Verification items for the finished model (mm, model axes). Face numbers are marked on the shaded views. A direction names the side the tool comes from. Give positions to 0.01 mm unless a question says otherwise; leave off trailing zeros. Write each loop counter-clockwise with the first axis right and the second up, starting at its lowest first coordinate (ties: lowest second). Pieces come first, ordered by that corner, then holes. Notation, with made-up numbers: (81, 23.25) -> (86, 23.25) arc R22 ccw to (86, 29.25) -> close; hole circle Ø6 at (-9.5, 11). An arc over 180 degrees is marked (long way). Answer as CSV lines item,"result". Start each with the question number.
1) Sectioned sample at C-C on y = 18. Record the cut outline in (x, z), and give its area (3 significant figures).
2) Tool access check on the marked faces 5, 6 and 7. Record the directions out of +Z, -Z, +X, -X, +Y, -Y that give a thin tool (end or side, any length) a straight path to the whole face; none if there is none.
3) Gauge pin test, flat ends, axial feed: pin 1 Ø10 at (x, y) = (-4.5, 21) entering from +Z; pin 2 Ø1.5 at (x, z) = (5, 2) entering from +Y; pin 3 Ø9 at (x, y) = (0, 23.5) entering from -Z. Record the tip position at first contact, or that the pin passes through.
4) Mould release check, pull along Z, two halves, no side actions. Record for the marked faces 1, 2, 3 and 4: released by +Z, released by -Z, zero draft, split by the parting line, or undercut.
5) Sectioned sample at B-B on z = 4.5. Record the cut outline in (x, y).
6) Sectioned sample at A-A on y = -0.5. Record the cut outline in (x, z), and give its area (3 significant figures).
7) Material ranges on L1, parallel to Z at x = 3, y = 2.5; L2, parallel to Z at x = -2, y = 41; L3, parallel to Y at x = -11.5, z = 13, recorded low to high.
```python
from build123d import *

# Parameters (mm, degrees)
F0_W     = 31.75
F0_H     = 25.4
F1_DEPTH = 3.81
F2_W     = 31.75
F2_H     = 3.81
F3_DEPTH = 3.81
F5_W     = 31.75
F5_H     = 5.08
F6_DEPTH = 31.75
F7_R     = 8.5850562929
F8_DEPTH = 10.161
F9_R     = 15.875
F10_R    = 15.87499
F11_R    = 1.27
F12_R    = 2.53999


# Not quite as in the source:
# - a fillet or chamfer is up to 0.001 mm smaller than in the source, because OpenCascade refuses the exact size


with BuildPart() as f1:
    # F0 (on Top) → F1 (new body)
    with BuildSketch(Plane.XY):
        with Locations((1.8298272586, 1.9303451554)):
            Rectangle(F0_W, F0_H)
    extrude(amount=F1_DEPTH)

    # F2 (on face) → F3 (join)
    with BuildSketch(Plane.XY.offset(3.81)):
        with Locations((1.8298272586, 12.7253451554)):
            Rectangle(F2_W, F2_H)
    extrude(amount=F3_DEPTH)

    # F4: F1 across face


with BuildPart() as f1_1:
    add(f1.part)
    add(f1.part.mirror(Plane(origin=(1.8298272586, 12.7253451554, 7.62), x_dir=(1, 0, 0), z_dir=(0, 0, 1))))

    # F5 (on face) → F6 (join)
    with BuildSketch(Plane(origin=(0, 14.6303451554, 0), x_dir=(-1, 0, 0), z_dir=(0, 1, 0))):
        with Locations((-1.8298272586, 7.62)):
            Rectangle(F5_W, F5_H)
    extrude(amount=F6_DEPTH)

    # F7 (on face) → F8 (cut, through all)
    with BuildSketch(Plane(origin=(0, 0, 5.08), x_dir=(1, 0, 0), z_dir=(0, 0, -1))):
        with Locations((1.8298272586, -30.5053451554)):
            Circle(F7_R)
    extrude(amount=-F8_DEPTH, mode=Mode.SUBTRACT)

    # F9
    f9_edges = [f1_1.edges().sort_by_distance(p)[0] for p in [
        (17.704827, 46.380345, 7.62),
    ]]
    fillet(f9_edges, radius=F9_R)

    # F10 (radius 15.875 in the source; OpenCascade refuses exactly that, so slightly less here)
    f10_edges = [f1_1.edges().sort_by_distance(p)[0] for p in [
        (-14.045173, 46.380345, 7.62),
    ]]
    fillet(f10_edges, radius=F10_R)

    # F11
    f11_edges = [f1_1.edges().sort_by_distance(p)[0] for p in [
        (-14.045173, -10.769655, 13.335),
        (-14.045173, 0.025345, 11.43),
        (-14.045173, 1.930345, 15.24),
        (-14.045173, 0.025345, 3.81),
        (-14.045173, 1.930345, 0),
        (-14.045173, 10.820345, 7.62),
        (-14.045173, 22.56785, 10.16),
        (-14.045173, 22.56785, 5.08),
        (1.829827, 14.630345, 15.24),
        (-14.045173, 14.630345, 12.7),
        (-14.045173, 14.630345, 2.54),
        (1.829827, -10.769655, 3.81),
        (1.829827, -10.769655, 11.43),
        (1.829827, -10.769655, 0),
        (1.829827, -10.769655, 15.24),
        (17.704827, 1.930345, 15.24),
        (17.704827, 0.025345, 11.43),
        (17.704827, 0.025345, 3.81),
        (17.704827, 1.930345, 0),
        (17.704827, 14.630345, 2.54),
        (17.704827, 14.630345, 12.7),
        (17.704827, 10.820345, 7.62),
    ]]
    fillet(f11_edges, radius=F11_R)

    # F12 (radius 2.54 in the source; OpenCascade refuses exactly that, so slightly less here)
    f12_edges = [f1_1.edges().sort_by_distance(p)[0] for p in [
        (-6.755229, 30.505345, 10.16),
        (-6.755229, 30.505345, 5.08),
    ]]
    fillet(f12_edges, radius=F12_R)


solid = f1_1.part
```
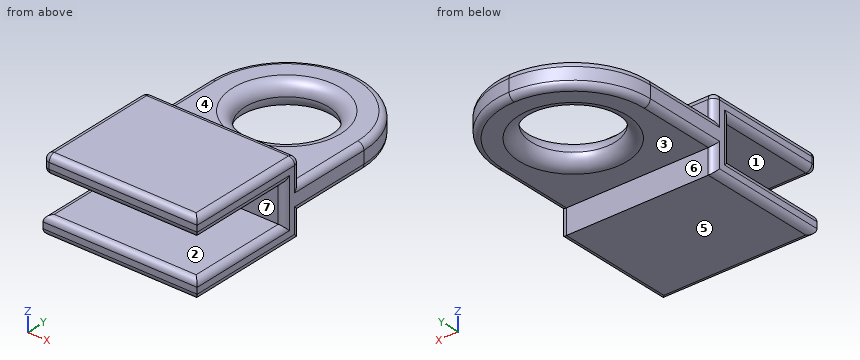
Ans:
1,outline,"(-14.05, 6.35) arc R1.27 ccw to (-12.78, 5.08) -> (16.43, 5.08) arc R1.27 ccw to (17.7, 6.35) -> (17.7, 8.89) arc R1.27 ccw to (16.43, 10.16) -> (-12.78, 10.16) arc R1.27 ccw to (-14.05, 8.89) -> close"
1,area,"160 mm²"
2,face 5,"-Z, +X, -X, +Y, -Y"
2,face 6,"-Z, +X, -X, +Y"
2,face 7,"+X, -X, -Y"
3,pin 1,"stops at z = 10.16"
3,pin 2,"stops at y = 14.63"
3,pin 3,"stops at z = 5.08"
4,face 1,"undercut"
4,face 2,"undercut"
4,face 3,"released by -Z"
4,face 4,"released by +Z"
5,outline,"(-14.05, 12.09) arc R1.27 ccw to (-12.78, 10.82) -> (16.43, 10.82) arc R1.27 ccw to (17.7, 12.09) -> (17.7, 13.36) arc R1.27 ccw to (16.43, 14.63) -> (-12.78, 14.63) arc R1.27 ccw to (-14.05, 13.36) -> close"
6,outline,"(-14.05, 1.27) arc R1.27 ccw to (-12.78, 0) -> (16.43, 0) arc R1.27 ccw to (17.7, 1.27) -> (17.7, 2.54) arc R1.27 ccw to (16.43, 3.81) -> (-12.78, 3.81) arc R1.27 ccw to (-14.05, 2.54) -> close; (-14.05, 12.7) arc R1.27 ccw to (-12.78, 11.43) -> (16.43, 11.43) arc R1.27 ccw to (17.7, 12.7) -> (17.7, 13.97) arc R1.27 ccw to (16.43, 15.24) -> (-12.78, 15.24) arc R1.27 ccw to (-14.05, 13.97) -> close"
6,area,"239 mm²"
7,L1,"z = 0 to 3.81, 11.43 to 15.24"
7,L2,"z = 5.08 to 10.16"
7,L3,"y = -10.77 to 14.63"
